```python
from build123d import *

# Parameters (mm, degrees)
SKETCH1_R           = 5.75
SKETCH1_R_2         = 4
BOSS_EXTRUDE1_DEPTH = 10
BOSS_EXTRUDE2_START = -3
SKETCH1_3_R         = 5.75
SKETCH1_3_R_2       = 3
SKETCH1_3_R_3       = 4
BOSS_EXTRUDE2_DEPTH = 3
BOSS_EXTRUDE3_START = -13
SKETCH1_4_R         = 3
SKETCH1_4_R_2       = 2
BOSS_EXTRUDE3_DEPTH = 13
BOSS_EXTRUDE4_START = -3
SKETCH1_5_R         = 7
SKETCH1_5_R_2       = 5.75
BOSS_EXTRUDE4_DEPTH = 3
FILLET1_R           = 10
CHAMFER1_SIZE       = 1


with BuildPart() as part:
    # Sketch1 → Boss-Extrude1 (new body)
    with BuildSketch(Plane.XY):
        Circle(SKETCH1_R)
        Circle(SKETCH1_R_2, mode=Mode.SUBTRACT)
    extrude(amount=BOSS_EXTRUDE1_DEPTH)

    # Sketch1<3> → Boss-Extrude2 (add)
    # profile 1 of 2: a face of its own
    with BuildSketch(Plane.XY.offset(BOSS_EXTRUDE2_START)):
        Circle(SKETCH1_3_R)
        Circle(SKETCH1_3_R_2, mode=Mode.SUBTRACT)
    # profile 2 of 2: a face of its own
    with BuildSketch(Plane.XY.offset(BOSS_EXTRUDE2_START)):
        Circle(SKETCH1_3_R_3)
        Circle(SKETCH1_3_R_2, mode=Mode.SUBTRACT)
    extrude(amount=BOSS_EXTRUDE2_DEPTH)

    # Sketch1<4> → Boss-Extrude3 (add)
    with BuildSketch(Plane.XY.offset(BOSS_EXTRUDE3_START)):
        Circle(SKETCH1_4_R)
        Circle(SKETCH1_4_R_2, mode=Mode.SUBTRACT)
    extrude(amount=BOSS_EXTRUDE3_DEPTH)

    # Sketch1<5> → Boss-Extrude4 (add)
    with BuildSketch(Plane.XY.offset(BOSS_EXTRUDE4_START)):
        Circle(SKETCH1_5_R)
        Circle(SKETCH1_5_R_2, mode=Mode.SUBTRACT)
    extrude(amount=BOSS_EXTRUDE4_DEPTH)

    # Fillet1
    # the kernel refuses this fillet: 10 mm, written as the material it takes off along each edge
    with BuildSketch(Plane(origin=(0, 0, 0), x_dir=(1, 0, 0), z_dir=(0, -1, 0))) as fillet1_piece_1:
        with BuildLine():
            CenterArc((12, -6), FILLET1_R, 143.130102354, 36.869897646)
            Line((2, -6), (1.8, -6))
            Line((1.8, -6), (1.8, 0))
            Line((1.8, 0), (2, 0.2))
            ThreePointArc((2, 0.2), (3, 0.2), (3.84, 0.12))
            Line((3.84, 0.12), (4, 0))
        make_face()
    revolve(axis=Axis((0, 0, 0), (0, 0, 1)), mode=Mode.SUBTRACT)

    # Chamfer1
    chamfer1_edges = [part.edges().sort_by_distance(p)[0] for p in [
        (-5.75, 0, 10),
    ]]
    chamfer(chamfer1_edges, length=CHAMFER1_SIZE)


solid = part.part
```
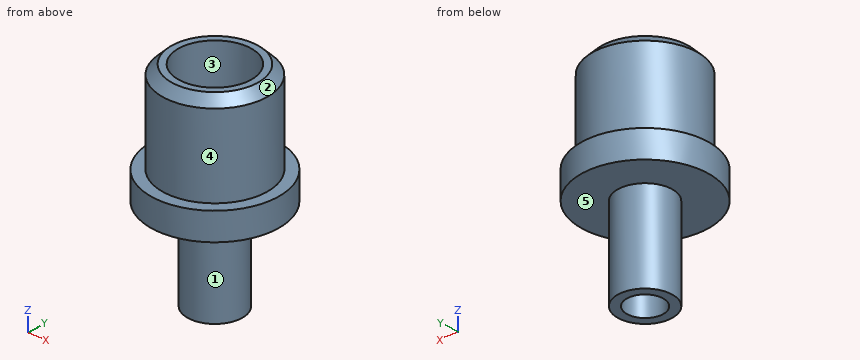
Design review of the part built by this model. Coordinates are the model's own, in mm. Face numbers are marked on the shaded views. A direction names the side the tool comes from. Give positions to 0.01 mm unless a question says otherwise; leave off trailing zeros. Loops run counter-clockwise (first coordinate to the right, second up) from the corner with the lowest first, then second, coordinate; pieces in that order, holes last. Notation, with made-up numbers: (33, 68.25) -> (62, 68.25) arc R18 cw to (62, 90.25) -> close; hole circle Ø8 at (63.5, 14). An arc over 180 degrees is marked (long way). One line per item, written item: value.
Q1. Machinability: for the marked faces 1 and 2, which of the approach directions +Z, -Z, +X, -X, +Y, -Y give a long, thin tool a straight path to every point of the face, cutting with its end or side? Answer none if there is none.
Numbers:
face 1: -Z
face 2: +Z
Q2. We need section A-A on x = 0. Give the boundary of the cut face in (y, z).
Numbers:
outline: (-7, -3) -> (-3, -3) -> (-3, -13) -> (-2, -13) -> (-2, -6) arc R10 ccw to (-4, 0) -> (-4, 10) -> (-4.75, 10) -> (-5.75, 9) -> (-5.75, 0) -> (-7, 0) -> close; (2, -13) -> (3, -13) -> (3, -3) -> (7, -3) -> (7, 0) -> (5.75, 0) -> (5.75, 9) -> (4.75, 10) -> (4, 10) -> (4, 0) arc R10 ccw to (2, -6) -> close
Q3. Draft analysis for pull direction X (two halves, no side actions). For the marked faces 3, 4 and 5, state which applies: pulls with the +X half, pulls with the -X half, needs draft (parallel to the pull), parting line crosses it, or undercut.
Numbers:
face 3: undercut
face 4: parting line crosses it
face 5: needs draft
Q4. We need section D-D on z = -7. Give the boundary of the cut face in (x, y), and give its area (3 significant figures).
Numbers:
outline: circle Ø6 at (0, 0); hole circle Ø4 at (0, 0)
area: 15.7 mm^2
Q5. We need section B-B on z = 5. Give the boundary of the cut face in (x, y).
Numbers:
outline: circle Ø11.5 at (0, 0); hole circle Ø8 at (0, 0)
Q6. For pin 1 Ø4 at (x, z) = (-3.5, 7.5) entering from +Y; pin 2 Ø1.5 at (x, y) = (-2.5, 5) entering from +Z; pin 3 Ø8 at (y, z) = (-3.5, -9) entering from -X; pin 4 Ø1.5 at (x, z) = (5.5, -4) entering from +Y, all flat-tipped, find the tip position at first contact; note any pin that passes through.
Numbers:
pin 1: stops at y = 5.55
pin 2: stops at z = 9.91
pin 3: stops at x = -3
pin 4: passes through
Q7. We need section C-C on x = -6. Give the boundary of the cut face in (y, z).
Numbers:
outline: (-3.61, -3) -> (3.61, -3) -> (3.61, 0) -> (-3.61, 0) -> close
Q8. For L1, parallel to Y at x = 0, z = -9.5; L2, parallel to Y at x = 0, z = 2.5; L3, parallel to Z at x = -4.5, y = -5, list the stretches that pass through material, from the lowest coordinate up.
Numbers:
L1: y = -3 to -2, 2 to 3
L2: y = -5.75 to -4, 4 to 5.75
L3: z = -3 to 0
